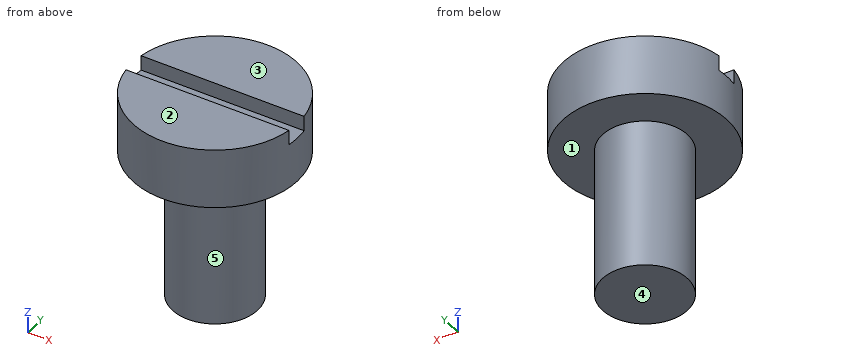
Solid Edge part; units mm, degrees
sketch "Sketch1" plane through (0, 0, 0) normal (0, 0, 1) x (1, 0, 0)
  circle A0 centre (0, 0) radius 1.425
extrude "Protrusion1" add sketch "Sketch1" against normal blind 5
sketch "Sketch2" plane through (0, 0, 0) normal (0, 0, 1) x (1, 0, 0)
  circle A0 centre (0, 0) radius 2.75
extrude "ExtrudedProtrusion_2" add sketch "Sketch2" along normal blind 2
sketch "Sketch3" plane through (0, 0, 2) normal (0, 0, 1) x (1, 0, 0)
  line L0 (3.6964, 0.4) -> (-3.6964, 0.4)
  line L1 (-3.6964, 0.4) -> (-3.6964, -0.4)
  line L2 (-3.6964, -0.4) -> (3.6964, -0.4)
  line L3 (3.6964, -0.4) -> (3.6964, 0.4)
extrude "ExtrudedCutout_1" cut sketch "Sketch3" against normal blind 0.5
properties material "Graphite"
The listing builds one solid part. Answer for the finished solid, in the listing's coordinates (mm). Face numbers are marked on the shaded views. A direction names the side the tool comes from. Coordinates: 2 decimals unless noted, no trailing zeros. Write each loop counter-clockwise with the first axis right and the second up, starting at its lowest first coordinate (ties: lowest second). Pieces come first, ordered by that corner, then holes. Notation, with made-up numbers: (44.5, 75.25) - (89.5, 75.25) arc R16 ccw to (89.5, 103.25) - close; hole circle Ø5 at (87, 57). An arc over 180 degrees is marked (long way). Return JSON: item names as keys, results as strings.
1. The part is cut by section C-C on z = -3.5. Determine the outline of the cut face in (x, y) (3 decimals).
Final values:
{"outline": "circle Ø2.85 at (0, 0)"}
2. The part is cut by section B-B on x = 0. Determine the outline of the cut face in (y, z) (3 decimals), then the cut area to 4 significant figures.
Final values:
{"outline": "(-2.75, 0) - (-1.425, 0) - (-1.425, -5) - (1.425, -5) - (1.425, 0) - (2.75, 0) - (2.75, 2) - (0.4, 2) - (0.4, 1.5) - (-0.4, 1.5) - (-0.4, 2) - (-2.75, 2) - close", "area": "24.85 mm^2"}
3. Which of the six approach directions +Z, -Z, +X, -X, +Y, -Y give full straight-line access (tool end or side, diameter ignored) to the marked faces 1 and 2?
Final values:
{"face 1": "-Z", "face 2": "+Z, +X, -X, +Y, -Y"}
4. For a pull along Z with two mould halves and no side action, classify the marked faces 3, 4 and 5 as +Z half, -Z half, draft (parallel to the pull), parting line (faces both ways), or undercut.
Final values:
{"face 3": "+Z half", "face 4": "-Z half", "face 5": "draft"}
5. Consider line 1 along Z through (x, y) = (1.45, 1.3); line 2 along Y through (x, z) = (-0.05, -1); line 3 along Y through (x, z) = (-0.1, 0.25). Determine where each line is inside the solid, lowest interval first.
Final values:
{"line 1": "0 to 2", "line 2": "-1.42 to 1.42", "line 3": "-2.75 to 2.75"}
6. Each of these flat-tipped pins is pushed along its axis until it touches: pin 1 Ø3 at (x, z) = (0, -4) entering from -Y (3 decimals); pin 2 Ø2 at (y, z) = (-1.5, -4) entering from -X. Where does it stop, or does it pass through?
Final values:
{"pin 1": "y = -1.425", "pin 2": "x = -1.33"}
7. The part is cut by section D-D on y = -0.7. Determine the outline of the cut face in (x, z).
Final values:
{"outline": "(-2.66, 0) - (-1.24, 0) - (-1.24, -5) - (1.24, -5) - (1.24, 0) - (2.66, 0) - (2.66, 2) - (-2.66, 2) - close"}
8. The part is cut by section A-A on y = 0. Determine the outline of the cut face in (x, z) (3 decimals).
Final values:
{"outline": "(-2.75, 0) - (-1.425, 0) - (-1.425, -5) - (1.425, -5) - (1.425, 0) - (2.75, 0) - (2.75, 1.5) - (-2.75, 1.5) - close"}
